```python
from build123d import *

# Parameters (mm, degrees)
SKETCH1_R           = 75
BOSS_EXTRUDE1_DEPTH = 2
SKETCH2_R           = 31
SKETCH2_R_2         = 29
EXTRUDE_THIN1_DEPTH = 8
SKETCH3_R           = 20
CUT_EXTRUDE1_DEPTH  = 3
SKETCH4_R           = 22
SKETCH4_R_2         = 20
EXTRUDE_THIN2_DEPTH = 10
FILLET1_R           = 5


with BuildPart() as part:
    # Sketch1 → Boss-Extrude1 (new body)
    with BuildSketch(Plane(origin=(0, 0, 0), x_dir=(1, 0, 0), z_dir=(0, 1, 0))):
        Circle(SKETCH1_R)
    extrude(amount=BOSS_EXTRUDE1_DEPTH)

    # Sketch2 → Extrude-Thin1 (add)
    with BuildSketch(Plane.XZ):
        Circle(SKETCH2_R)
        Circle(SKETCH2_R_2, mode=Mode.SUBTRACT)
    extrude(amount=EXTRUDE_THIN1_DEPTH)

    # Sketch3 → Cut-Extrude1 (cut, through all)
    with BuildSketch(Plane.XZ):
        Circle(SKETCH3_R)
    extrude(amount=-CUT_EXTRUDE1_DEPTH, mode=Mode.SUBTRACT)

    # Sketch4 → Extrude-Thin2 (add)
    with BuildSketch(Plane(origin=(0, 2, 0), x_dir=(1, 0, 0), z_dir=(0, 1, 0))):
        Circle(SKETCH4_R)
        Circle(SKETCH4_R_2, mode=Mode.SUBTRACT)
    extrude(amount=EXTRUDE_THIN2_DEPTH)

    # Fillet1
    fillet1_edges = [part.edges().sort_by_distance(p)[0] for p in [
        (-22, 2, 0),
    ]]
    fillet(fillet1_edges, radius=FILLET1_R)


solid = part.part
```
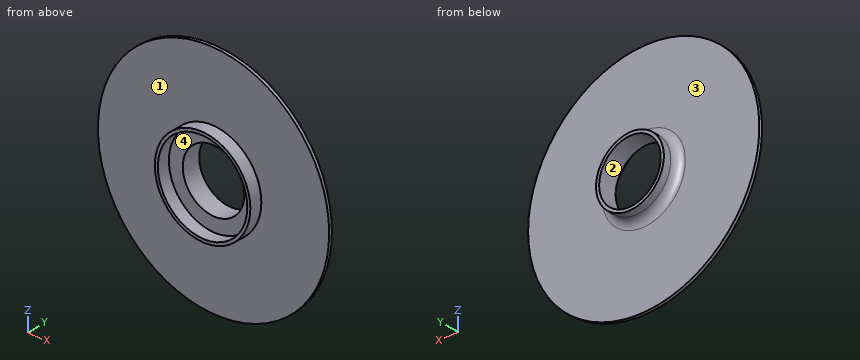
Model file for the job. Use its own axes, mm. Face numbers are marked on the shaded views. A direction names the side the tool comes from. Give positions to 0.01 mm unless a question says otherwise; leave off trailing zeros. Write each loop counter-clockwise with the first axis right and the second up, starting at its lowest first coordinate (ties: lowest second). Pieces come first, ordered by that corner, then holes. Notation, with made-up numbers: M 67.25,17.25 L 97.25,17.25 A18 cw 97.25,30.25 Z; hole C -11.75,55.5 d3. An arc over 180 degrees is marked long. Use a Markdown table: item, result.
1) Cut at D-D (y = 10.25). List the corners of the cut face in (x, z), and give its area (3 significant figures).
Responses:
| item | result |
|---|---|
| outline | C 0,0 d44; hole C 0,0 d40 |
| area | 264 mm2 |
2) Drill centre lines: line 1 (Z direction, x = 0.5, y = 7); line 2 (Z direction, x = 0, y = -2.25); line 3 (Y direction, x = 26, z = 13). Where is each one in solid material? Low to high. Write a range as from..to.
Responses:
| item | result |
|---|---|
| line 1 | z = -21.99..-19.99, 19.99..21.99 |
| line 2 | z = -31..-29, 29..31 |
| line 3 | y = -8..2 |
3) Cut at B-B (x = 0). List the corners of the cut face in (y, z).
Responses:
| item | result |
|---|---|
| outline | M -8,-31 L 0,-31 L 0,-75 L 2,-75 L 2,-27 A5 cw 7,-22 L 12,-22 L 12,-20 L 0,-20 L 0,-29 L -8,-29 Z; M -8,29 L 0,29 L 0,20 L 12,20 L 12,22 L 7,22 A5 cw 2,27 L 2,75 L 0,75 L 0,31 L -8,31 Z |
4) Cut at A-A (z = 0). List the corners of the cut face in (x, y), and give its area (3 significant figures).
Responses:
| item | result |
|---|---|
| outline | M -75,0 L -31,0 L -31,-8 L -29,-8 L -29,0 L -20,0 L -20,12 L -22,12 L -22,7 A5 cw -27,2 L -75,2 Z; M 20,0 L 29,0 L 29,-8 L 31,-8 L 31,0 L 75,0 L 75,2 L 27,2 A5 cw 22,7 L 22,12 L 20,12 Z |
| area | 303 mm2 |
5) Cut at C-C (y = -4.5). List the corners of the cut face in (x, z), and give its area (3 significant figures).
Responses:
| item | result |
|---|---|
| outline | C 0,0 d62; hole C 0,0 d58 |
| area | 377 mm2 |
6) Pin check, flat tips, straight feed: pin 1 (10 mm diameter, centred on y = -1.5, z = -23.5, fed in from -X); pin 2 (12 mm diameter, centred on x = 56, z = -20.5, fed in from +Y); pin 3 (3 mm diameter, centred on y = 2, z = -17.5, fed in from +X). Stop position of each tip, or through.
Responses:
| item | result |
|---|---|
| pin 1 | stops at x = -72.62 |
| pin 2 | stops at y = 2 |
| pin 3 | stops at x = 73.27 |
7) Pull direction Z, two halves, no side cores. Call the marked faces 3 and 4: +Z half, -Z half, draft (parallel to the pull), parting line (faces both ways), or undercut.
Responses:
| item | result |
|---|---|
| face 3 | draft |
| face 4 | undercut |
8) Tool access for the marked faces 1 and 2: list every direction of +Z, -Z, +X, -X, +Y, -Y with a clear straight run to the whole face (end or side of a thin tool).
Responses:
| item | result |
|---|---|
| face 1 | -Y |
| face 2 | +Y, -Y |
